Autodesk Inventor part; units mm, degrees
ref_plane "YZ Plane" through (0, 0, 0) normal (1, 0, 0) x (0, 1, 0)
ref_plane "XZ Plane" through (0, 0, 0) normal (0, 1, 0) x (-1, 0, 0)
ref_plane "XY Plane" through (0, 0, 0) normal (0, 0, 1) x (1, 0, 0)
sketch "Sketch3" plane through (0, 0, 1) normal (0, 0, 1) x (1, 0, 0)
  line L0 (-22.5, 27.5) -> (-12.5, 27.5)
  line L1 (-7.5, 22.5) -> (-7.5, 12.5)
  line L2 (-12.5, 7.5) -> (-22.5, 7.5)
  line L3 (-27.5, 12.5) -> (-27.5, 22.5)
  line L4 (-27.5, 27.5) -> (-7.5, 7.5) construction
  line L5 (-7.5, 27.5) -> (-27.5, 7.5) construction
  line L6 (-11.1923, 0) -> (11.1923, 0)
  line L7 (0, 8.4231) -> (0, -8.4231)
  arc A0 (-22.5, 27.5) -> (-27.5, 22.5) centre (-22.5, 22.5) ccw
  arc A1 (-7.5, 22.5) -> (-12.5, 27.5) centre (-12.5, 22.5) ccw
  arc A2 (-12.5, 7.5) -> (-7.5, 12.5) centre (-12.5, 12.5) ccw
  arc A3 (-27.5, 12.5) -> (-22.5, 7.5) centre (-22.5, 12.5) ccw
  line L8 (22.5, 27.5) -> (12.5, 27.5)
  line L9 (7.5, 22.5) -> (7.5, 12.5)
  line L10 (12.5, 7.5) -> (22.5, 7.5)
  line L11 (27.5, 12.5) -> (27.5, 22.5)
  line L12 (27.5, 27.5) -> (7.5, 7.5) construction
  line L13 (7.5, 27.5) -> (27.5, 7.5) construction
  arc A4 (27.5, 22.5) -> (22.5, 27.5) centre (22.5, 22.5) ccw
  arc A5 (12.5, 27.5) -> (7.5, 22.5) centre (12.5, 22.5) ccw
  arc A6 (7.5, 12.5) -> (12.5, 7.5) centre (12.5, 12.5) ccw
  arc A7 (22.5, 7.5) -> (27.5, 12.5) centre (22.5, 12.5) ccw
  line L14 (-22.5, -27.5) -> (-12.5, -27.5)
  line L15 (-7.5, -22.5) -> (-7.5, -12.5)
  line L16 (-12.5, -7.5) -> (-22.5, -7.5)
  line L17 (-27.5, -12.5) -> (-27.5, -22.5)
  line L18 (-27.5, -27.5) -> (-7.5, -7.5) construction
  line L19 (-7.5, -27.5) -> (-27.5, -7.5) construction
  arc A8 (-27.5, -22.5) -> (-22.5, -27.5) centre (-22.5, -22.5) ccw
  arc A9 (-12.5, -27.5) -> (-7.5, -22.5) centre (-12.5, -22.5) ccw
  arc A10 (-7.5, -12.5) -> (-12.5, -7.5) centre (-12.5, -12.5) ccw
  arc A11 (-22.5, -7.5) -> (-27.5, -12.5) centre (-22.5, -12.5) ccw
  line L20 (7.5, -22.5) -> (7.5, -12.5)
  arc A12 (12.5, -7.5) -> (7.5, -12.5) centre (12.5, -12.5) ccw
  arc A13 (7.5, -22.5) -> (12.5, -27.5) centre (12.5, -22.5) ccw
  line L21 (22.5, -27.5) -> (12.5, -27.5)
  line L22 (12.5, -7.5) -> (22.5, -7.5)
  line L23 (27.5, -27.5) -> (7.5, -7.5) construction
  line L24 (7.5, -27.5) -> (27.5, -7.5) construction
  arc A14 (27.5, -12.5) -> (22.5, -7.5) centre (22.5, -12.5) ccw
  line L25 (27.5, -12.5) -> (27.5, -22.5)
  arc A15 (22.5, -27.5) -> (27.5, -22.5) centre (22.5, -22.5) ccw
  point P0 (0, 0)
  point P1 (-17.5, 17.5)
  point P2 (0, 0)
  point P3 (17.5, 17.5)
  point P4 (-17.5, -17.5)
  point P5 (17.5, -17.5)
  dimension "d29" = 20
  dimension "d30" = 15
  dimension "d31" = 15
  dimension "d32" = 20
  dimension "d33" = 5
sketch "Sketch1" plane through (0, 0, 0) normal (0, 0, 1) x (1, 0, 0)
  line L0 (-36, 20) -> (36, 20)
  line L1 (36, 20) -> (36, -20)
  line L2 (36, -20) -> (-36, -20)
  line L3 (-36, -20) -> (-36, 20)
  line L4 (-36, 20) -> (36, -20) construction
  line L5 (36, 20) -> (-36, -20) construction
  point P0 (0, 0)
  dimension "d0" = 40
  dimension "d1" = 72
extrude "Plate1" add sketch "Sketch1" along normal blind 1
sketch "Sketch2" plane through (0, 0, 1) normal (0, 0, 1) x (1, 0, 0)
  line L0 (-36, 20) -> (36, 20)
  line L1 (-46, -5) -> (-36, -5)
  line L2 (-36, -5) -> (-36, 5)
  line L3 (-36, 5) -> (-46, 5)
  line L4 (-46, 5) -> (-46, -5)
  line L5 (-46, -5) -> (-36, 5) construction
  line L6 (-36, -5) -> (-46, 5) construction
  line L7 (0, 0) -> (0, 7.0571)
  line L8 (0, 0) -> (6.6312, 0)
  line L9 (-36, -20) -> (-36, 20)
  line L10 (46, -5) -> (36, -5)
  line L11 (36, -5) -> (36, 5)
  line L12 (36, 5) -> (46, 5)
  line L13 (46, 5) -> (46, -5)
  line L14 (46, -5) -> (36, 5) construction
  line L15 (36, -5) -> (46, 5) construction
  circle A0 centre (-42, 0) radius 1.6
  circle A1 centre (42, 0) radius 1.6
  line L16 (36, -20) -> (-36, -20)
  line L17 (-5, -30) -> (5, -30)
  line L18 (5, -30) -> (5, -20)
  line L19 (5, -20) -> (-5, -20)
  line L20 (-5, -20) -> (-5, -30)
  line L21 (-5, -30) -> (5, -20) construction
  line L22 (5, -30) -> (-5, -20) construction
  circle A2 centre (0, -26) radius 1.6
  line L23 (-5, 30) -> (5, 30)
  line L24 (5, 30) -> (5, 20)
  line L25 (5, 20) -> (-5, 20)
  line L26 (-5, 20) -> (-5, 30)
  line L27 (-5, 30) -> (5, 20) construction
  line L28 (5, 30) -> (-5, 20) construction
  circle A3 centre (0, 26) radius 1.6
  point P0 (-41, 0)
  point P1 (41, 0)
  point P2 (0, -25)
  point P3 (0, 25)
  dimension "d5" = 10
  dimension "d6" = 10
  dimension "d10" = 3.2
  dimension "d12" = 4
  dimension "d18" = 3.2
  dimension "d19" = 10
  dimension "d20" = 10
  dimension "d21" = 4
sheet face with bend "Face2" sketch "Sketch2" thickness 1 toward (0, 0, -1) bend radius 1
bend "Bend1"
sketch "Sketch4" plane through (0, 0, 1) normal (0, 0, 1) x (1, 0, 0)
  line L0 (-22.5, 12.5) -> (-12.5, 12.5)
  line L1 (-7.5, 7.5) -> (-7.5, -7.5)
  line L2 (-12.5, -12.5) -> (-22.5, -12.5)
  line L3 (-27.5, -7.5) -> (-27.5, 7.5)
  line L4 (-27.5, 12.5) -> (-7.5, -12.5) construction
  line L5 (-7.5, 12.5) -> (-27.5, -12.5) construction
  line L6 (0, 16.1761) -> (0, -17.081)
  arc A0 (-22.5, 12.5) -> (-27.5, 7.5) centre (-22.5, 7.5) ccw
  arc A1 (-7.5, 7.5) -> (-12.5, 12.5) centre (-12.5, 7.5) ccw
  arc A2 (-12.5, -12.5) -> (-7.5, -7.5) centre (-12.5, -7.5) ccw
  arc A3 (-27.5, -7.5) -> (-22.5, -12.5) centre (-22.5, -7.5) ccw
  line L7 (22.5, 12.5) -> (12.5, 12.5)
  line L8 (7.5, 7.5) -> (7.5, -7.5)
  line L9 (12.5, -12.5) -> (22.5, -12.5)
  line L10 (27.5, -7.5) -> (27.5, 7.5)
  line L11 (27.5, 12.5) -> (7.5, -12.5) construction
  line L12 (7.5, 12.5) -> (27.5, -12.5) construction
  arc A4 (27.5, 7.5) -> (22.5, 12.5) centre (22.5, 7.5) ccw
  arc A5 (12.5, 12.5) -> (7.5, 7.5) centre (12.5, 7.5) ccw
  arc A6 (7.5, -7.5) -> (12.5, -12.5) centre (12.5, -7.5) ccw
  arc A7 (22.5, -12.5) -> (27.5, -7.5) centre (22.5, -7.5) ccw
  point P0 (0, 0)
  point P1 (-17.5, 0)
  point P2 (17.5, 0)
  dimension "d36" = 20
  dimension "d37" = 25
  dimension "d38" = 5
  dimension "d39" = 15
extrude "Cut2" cut sketch "Sketch4" against normal blind 1
equation "\"d40\" = 厚度"
equation "\"d2\" = 厚度"
equation "\"d13\" = 折彎半徑"
equation "\"d14\" = 折彎離隙寬度"
equation "\"d16\" = 最小剩餘"
equation "\"d15\" = 折彎離隙深度"
equation "\"d17\" = 轉移半徑"
equation "\"折彎半徑\" = 厚度"
equation "\"折彎離隙寬度\" = 厚度"
equation "\"折彎離隙深度\" = 0.5 * 厚度"
equation "\"轉角離隙大小\" = 4 * 厚度"
equation "\"最小剩餘\" = 2 * 厚度"
equation "\"轉移半徑\" = 折彎半徑"
equation "\"Jacobi半徑大小\" = 折彎半徑"
equation "\"間隙大小\" = 厚度"
properties part number "battery_box_5V_top" material "Aluminum"
Verification items for the finished model (mm, model axes). A direction names the side the tool comes from. Coordinates: 2 decimals unless noted, no trailing zeros. Write each loop counter-clockwise with the first axis right and the second up, starting at its lowest first coordinate (ties: lowest second). Pieces come first, ordered by that corner, then holes. Notation, with made-up numbers: (77, 39.25) -> (106, 39.25) arc R30 cw to (106, 73.25) -> close; hole circle Ø1 at (-9, 42). An arc over 180 degrees is marked (long way). One line per item, written item: value. Start each with the question number.
Q1. Thickness scan on L1, parallel to Y at x = 0, z = 0.45; L2, parallel to Y at x = 17, z = 0.85; L3, parallel to X at y = 9, z = 0.8. Record the ranges inside material, lowest first. Write a range as from..to.
Q2. Access from +Z, -Z, +X, -X, +Y, -Y to the whole of each face (thin tool, end or side, straight path). Record for faces 1 (the flat face through (-1, -6, 0)), 2 (the cylindrical face through (-8.93, 11, 0.51)).
Q3. Cross-section at C-C on y = 0. Enter the section's corners in (x, z), and give its area (3 significant figures).
Q4. Cross-section at D-D on x = 0. Enter the section's corners in (y, z), and give its area (3 significant figures).
Q5. Cross-section at B-B on y = 6.5. Enter the section's corners in (x, z), and give its area (3 significant figures).
Q6. Cross-section at A-A on x = -9.5. Enter the section's corners in (y, z), and give its area (3 significant figures).
Q7. Go/stop test with flat-tipped pins: P1, Ø0.5, axis at x = 40, z = 0.5, coming from the -Y side; P2, Ø0.5, axis at x = -18, z = 0.5, coming from the +Y side; P3, Ø0.5, axis at y = -11.5, z = 0.5, coming from the -X side; P4, Ø3, axis at x = 0, y = -26, coming from the +Z side. Record where each tip stops, or that it passes through.
Checked values:
1. L1: y = -30..-27.6, -24.4..24.4, 27.6..30
1. L2: y = -20..-12.5, 12.5..20
1. L3: x = -36..-27.27, -7.73..7.73, 27.27..36
2. face 1: -Z, +X, -X, +Y, -Y
2. face 2: +Z, -Z
3. outline: (-46, 0) -> (-43.6, 0) -> (-43.6, 1) -> (-46, 1) -> close; (-40.4, 0) -> (-27.5, 0) -> (-27.5, 1) -> (-40.4, 1) -> close; (-7.5, 0) -> (7.5, 0) -> (7.5, 1) -> (-7.5, 1) -> close; (27.5, 0) -> (40.4, 0) -> (40.4, 1) -> (27.5, 1) -> close; (43.6, 0) -> (46, 0) -> (46, 1) -> (43.6, 1) -> close
3. area: 45.6 mm²
4. outline: (-30, 0) -> (-27.6, 0) -> (-27.6, 1) -> (-30, 1) -> close; (-24.4, 0) -> (24.4, 0) -> (24.4, 1) -> (-24.4, 1) -> close; (27.6, 0) -> (30, 0) -> (30, 1) -> (27.6, 1) -> close
4. area: 53.6 mm²
5. outline: (-36, 0) -> (-27.5, 0) -> (-27.5, 1) -> (-36, 1) -> close; (-7.5, 0) -> (7.5, 0) -> (7.5, 1) -> (-7.5, 1) -> close; (27.5, 0) -> (36, 0) -> (36, 1) -> (27.5, 1) -> close
5. area: 32.0 mm²
6. outline: (-20, 0) -> (-11.5, 0) -> (-11.5, 1) -> (-20, 1) -> close; (11.5, 0) -> (20, 0) -> (20, 1) -> (11.5, 1) -> close
6. area: 17.0 mm²
7. P1: stops at y = -5
7. P2: stops at y = 20
7. P3: stops at x = -36
7. P4: passes through
